from build123d import *

# Parameters (mm, degrees)
CYLINDER001_R     = 1
CYLINDER001_DEPTH = 3.5
BOX_W             = 13.5
BOX_H             = 6
BOX_DEPTH         = 0.5
CYLINDER_W        = 4
CYLINDER_H        = 13.5
CYLINDER_ANGLE    = 180


with BuildPart() as cylinder001:
    # Cylinder001 → Cylinder001 (new body)
    with BuildSketch(Plane(origin=(3.12, 3, 1), x_dir=(1, 0, 0), z_dir=(0, 0, 1))):
        Circle(CYLINDER001_R)
    extrude(amount=CYLINDER001_DEPTH)


with BuildPart() as cube:
    # Box → Box (new body)
    with BuildSketch(Plane.XY):
        with Locations((6.75, 3)):
            Rectangle(BOX_W, BOX_H)
    extrude(amount=BOX_DEPTH)


with BuildPart() as obj1:
    # Cylinder → Cylinder (revolve)
    with BuildSketch(Plane(origin=(0, 3, 0.5), x_dir=(0, 1, 0), z_dir=(0, 0, -1))):
        with Locations((2, 6.75)):
            Rectangle(CYLINDER_W, CYLINDER_H)
    revolve(axis=Axis((0, 3, 0.5), (1, 0, 0)), revolution_arc=CYLINDER_ANGLE)

    # Fusion: union Cube
    add(cube.part)

    # Cut: cut Cylinder001
    add(cylinder001.part, mode=Mode.SUBTRACT)


solid = obj1.part
Could you check a few things on this model? Use its own coordinates, in mm. A direction names the side the tool comes from. Give positions to 0.01 mm unless a question says otherwise; leave off trailing zeros. Order: outer loops, then holes, each group sorted by start corner. A loop starts at its lowest first (then second) coordinate and runs counter-clockwise, first axis right, second up.
Item 1: For faces 1 (the face through (7, 3, 0)), 2 (the face through (6.8, -0.5, 0.5)), 3 (the face through (3, 3, 1)), which set-ups out of +Z, -Z, +X, -X, +Y, -Y let a thin tool reach every point of the face, with its end or its side?
Item 2: I need wall thicknesses on line 1 (X direction, y = 3, z = 2.7); line 2 (Y direction, x = 3.12, z = 3.15); line 3 (Y direction, x = 2.75, z = 1.3). Which ranges of each line are inside material? Lowest first, please.
Item 3: If we section it at B-B, the plane y = 3: Write out the boundary of the cut face in (x, z).
Item 4: If we mould it in two halves opening along X, with no side actions, what happens to faces 4 (the face through (6.8, 6.5, 0.5)), 5 (the face through (13.5, 3, 2)), 6 (the face through (0, 3, 2)), 7 (the face through (2.383, 3.676, 2.726))? For each: pulls with the +X half, pulls with the -X half, needs draft (parallel to the pull), parting line crosses it, or undercut.
Item 5: I'm going to push flat-ended pins straight in: pin 1 (0.6 mm diameter, centred on x = 3.5, y = 3, fed in from +Z); pin 2 (1 mm diameter, centred on x = 11, z = 4, fed in from +Y). Where does each tip first touch, or does it pass through?
Item 6: If we section it at D-D, the plane x = 2.5: Write out the boundary of the cut face in (y, z), plus the area to 3 significant figures.
Item 7: If we section it at A-A, the plane x = 9.25: Write out the boundary of the cut face in (y, z), plus the area to 3 significant figures.
Item 8: If we section it at C-C, the plane z = 1.35: Write out the boundary of the cut face in (x, y), plus the area to 3 significant figures.
Values:
1. face 1: -Z, +X, -X, +Y, -Y
1. face 2: -Z, +X, -X, -Y
1. face 3: +Z
2. line 1: x = 0 to 2.12, 4.12 to 13.5
2. line 2: y = 0 to 2, 4 to 6
2. line 3: y = -0.92 to 2.07, 3.93 to 6.92
3. outline: (0, 0) - (13.5, 0) - (13.5, 4.5) - (4.12, 4.5) - (4.12, 1) - (2.12, 1) - (2.12, 4.5) - (0, 4.5) - close
4. face 4: needs draft
4. face 5: pulls with the +X half
4. face 6: pulls with the -X half
4. face 7: undercut
5. pin 1: stops at z = 1
5. pin 2: stops at y = 5.65
6. outline: (-1, 0.5) - (0, 0.5) - (0, 0) - (6, 0) - (6, 0.5) - (7, 0.5) arc R4 ccw to (3.78, 4.42) - (3.78, 1) - (2.22, 1) - (2.22, 4.42) arc R4 ccw to start
6. area: 22.7 mm2
7. outline: (-1, 0.5) - (0, 0.5) - (0, 0) - (6, 0) - (6, 0.5) - (7, 0.5) arc R4 ccw to start
7. area: 28.1 mm2
8. outline: (0, -0.91) - (13.5, -0.91) - (13.5, 6.91) - (0, 6.91) - close; hole circle Ø2 at (3.12, 3)
8. area: 102 mm2
